```python
from build123d import *

# Parameters (mm, degrees)
SKETCH1_R           = 4
BOSS_EXTRUDE1_DEPTH = 100
SKETCH2_R           = 7
BOSS_EXTRUDE2_DEPTH = 2
DOME1_FACE_RADIUS   = 7
DOME1_HEIGHT        = 4
FILLET1_R           = 0.1
CHAMFER1_SIZE       = 1


with BuildPart() as part:
    # Sketch1 → Boss-Extrude1 (new body)
    with BuildSketch(Plane(origin=(0, 0, 0), x_dir=(1, 0, 0), z_dir=(0, 1, 0))):
        with Locations(Location((0, 0, 0), (0, 0, 270))):
            Circle(SKETCH1_R)
    extrude(amount=BOSS_EXTRUDE1_DEPTH)

    # Sketch2 → Boss-Extrude2 (add)
    with BuildSketch(Plane(origin=(0, 100, 0), x_dir=(1, 0, 0), z_dir=(0, 1, 0))):
        with Locations(Location((0, 0, 0), (0, 0, 270))):
            Circle(SKETCH2_R)
    extrude(amount=BOSS_EXTRUDE2_DEPTH)

    # Dome1: an elliptical dome of height H over a round flat face of radius A is half a spheroid: the quarter ellipse of half axes A and H revolved about the face's axis
    with BuildSketch(Plane((0, 102, 0), x_dir=(0, 0, -1), z_dir=(1, 0, 0)), mode=Mode.PRIVATE) as dome1_quarter:
        Ellipse(DOME1_FACE_RADIUS, DOME1_HEIGHT)
        Rectangle(DOME1_FACE_RADIUS, DOME1_HEIGHT, align=(Align.MIN, Align.MIN), mode=Mode.INTERSECT)
    revolve(dome1_quarter.sketch, axis=Axis((0, 102, 0), (0, 1, 0)))

    # Fillet1
    fillet1_edges = [part.edges().sort_by_distance(p)[0] for p in [
        (0, 100, -4),
        (0, 100, -7),
    ]]
    fillet(fillet1_edges, radius=FILLET1_R)

    # Chamfer1
    chamfer1_edges = [part.edges().sort_by_distance(p)[0] for p in [
        (0, 0, -4),
    ]]
    chamfer(chamfer1_edges, length=CHAMFER1_SIZE)


solid = part.part
```
For this review, take the finished solid that the model builds, in its own axes (mm). A direction names the side the tool comes from. Round coordinates to 2 decimals unless told otherwise and drop trailing zeros. Write each loop counter-clockwise with the first axis right and the second up, starting at its lowest first coordinate (ties: lowest second). Pieces come first, ordered by that corner, then holes.
1) Insertion check: pin 1 Ø5 at (x, z) = (2, -4.5) entering from +Y; pin 2 Ø4 at (x, z) = (3.5, 1) entering from +Y; pin 3 Ø1 at (x, y) = (-4, 37) entering from +Z; pin 4 Ø1 at (x, y) = (5, 92.5) entering from -Z. Each pin has a flat end and moves straight along its axis. Give the tip position at first contact, or say it passes through.
Answer below:
pin 1: stops at y = 105.75
pin 2: stops at y = 105.89
pin 3: stops at z = 1.94
pin 4: passes through
2) Machinability: for faces 1 (the face through (-6.834, 101.037, -1.517)), 2 (the face through (-3.905, 49.758, -0.867)), which of the approach directions +Z, -Z, +X, -X, +Y, -Y give a long, thin tool a straight path to every point of the face, cutting with its end or side? Answer none if there is none.
Answer below:
face 1: +Y, -Y
face 2: -Y
3) Take a section at A-A on y = 34. Give the boundary of the cut face in (x, z), then the cut area to 3 significant figures.
Answer below:
outline: circle Ø8 at (0, 0)
area: 50.3 mm2
4) For line 1 along Y through (x, z) = (-0.5, 0); line 2 along X through (y, z) = (54, 3.25); line 3 along Z through (x, y) = (2.5, 41), list the stretches that pass through material, from the lowest coordinate up.
Answer below:
line 1: y = 0 to 105.99
line 2: x = -2.33 to 2.33
line 3: z = -3.12 to 3.12
